Could you check a few things on this model? Use its own coordinates, in mm. A direction names the side the tool comes from. Coordinates: 2 decimals unless noted, no trailing zeros. Loops run counter-clockwise (first coordinate to the right, second up) from the corner with the lowest first, then second, coordinate; pieces in that order, holes last.
1) Thinking about a two-plate mould opening in X: for faces 1 (the face through (-2, 0, -2)), 2 (the face through (4, 2, 0)), 3 (the face through (-0.225, -0.715, 2.24)), which applies, released by +X, released by -X, zero draft, split by the parting line, or undercut?
2) For faces 4 (the face through (13.17, 0.07, 1.5)), 5 (the face through (1, 0, 3)), 6 (the face through (4, -2, 0)), which set-ups out of +Z, -Z, +X, -X, +Y, -Y let a thin tool reach every point of the face, with its end or its side?
3) Will these pins go through, and if not, where does the flat tip stop? P1, Ø1.5, axis at y = -4, z = -0.5, coming from the +X side; P2, Ø1.5, axis at x = 2, z = 0, coming from the +Y side; P3, Ø2.5, axis at x = 3, z = -1, coming from the -Y side; P4, Ø1.5, axis at x = 4, y = -0.5, coming from the +Z side.
4) Imagine slicing it at D-D on x = -0.25. Please give me the cut outline in (y, z).
5) Imagine slicing it at B-B on z = 0. Please give me the cut outline in (x, y).
6) Imagine slicing it at A-A on y = 0. Give the number of separate pieces and of enclosed holes in the cut face, plus the area to 4 significant figures.
7) If I drill on line 1 along Z through (x, y) = (2, 1); line 2 along X through (y, z) = (0, -2.6); line 3 along X through (y, z) = (-3.5, 1), over which ranges is the centre line in solid material (lowest first)?
8) Imagine slicing it at C-C on z = 2.5. Please give me the cut outline in (x, y).
```python
from build123d import *

# Parameters (mm, degrees)
EXTRUDE_1_DEPTH     = 3
SKETCH_2_R          = 5
EXTRUDE_2_DEPTH     = 1.5
SKETCH_3_R          = 3.5
EXTRUDE_3_DEPTH     = 1
SKETCH_4_R          = 1.5
EXTRUDE_4_DEPTH     = 12
SKETCH_5_W          = 10
SKETCH_5_H          = 3
CUT_EXTRUDE_1_DEPTH = 22.313141486
CHAMFER_1_SIZE      = 0.5


with BuildPart() as part:
    # 草图1 → 凸台-拉伸1 (new, symmetric)
    with BuildSketch(Plane.XY):
        with BuildLine():
            Line((5, 2), (0, 2))
            ThreePointArc((0, 2), (1.414213562, 1.414213562), (2, 0))
            ThreePointArc((2, 0), (1.414213562, -1.414213562), (0, -2))
            Line((0, -2), (5, -2))
            Line((5, -2), (5, 2))
        make_face()
        with BuildLine():
            ThreePointArc((2, 0), (1.414213562, 1.414213562), (0, 2))
            Line((0, 2), (0, 0.75))
            ThreePointArc((0, 0.75), (0.530330086, 0.530330086), (0.75, 0))
            ThreePointArc((0.75, 0), (0.530330086, -0.530330086), (0, -0.75))
            Line((0, -0.75), (0, -2))
            ThreePointArc((0, -2), (1.414213562, -1.414213562), (2, 0))
        make_face()
        with BuildLine():
            Line((0, 0.75), (0, 2))
            ThreePointArc((0, 2), (-2, 0), (0, -2))
            Line((0, -2), (0, -0.75))
            ThreePointArc((0, -0.75), (-0.75, 0), (0, 0.75))
        make_face()
    extrude(amount=EXTRUDE_1_DEPTH, both=True)

    # 草图2 → 凸台-拉伸2 (add)
    with BuildSketch(Plane(origin=(5, 0, 0), x_dir=(0, 0, -1), z_dir=(1, 0, 0))):
        Circle(SKETCH_2_R)
    extrude(amount=EXTRUDE_2_DEPTH)

    # 草图3 → 凸台-拉伸3 (add)
    with BuildSketch(Plane(origin=(6.5, 0, 0), x_dir=(0, 0, -1), z_dir=(1, 0, 0))):
        Circle(SKETCH_3_R)
    extrude(amount=EXTRUDE_3_DEPTH)

    # 草图4 → 凸台-拉伸4 (add)
    with BuildSketch(Plane(origin=(7.5, 0, 0), x_dir=(0, 0, -1), z_dir=(1, 0, 0))):
        Circle(SKETCH_4_R)
    extrude(amount=EXTRUDE_4_DEPTH)

    # 草图5 → 切除-拉伸1 (cut, through all)
    with BuildSketch(Plane(origin=(0, 2, 0), x_dir=(1, 0, 0), z_dir=(0, 1, 0))):
        with Locations((-2, 0)):
            Rectangle(SKETCH_5_W, SKETCH_5_H)
    extrude(amount=-CUT_EXTRUDE_1_DEPTH, mode=Mode.SUBTRACT)

    # 倒角1
    chamfer_1_edges = [part.edges().sort_by_distance(p)[0] for p in [
        (19.5, 0, 1.5),
    ]]
    chamfer(chamfer_1_edges, length=CHAMFER_1_SIZE)


solid = part.part
```
Filled in:
1. face 1: released by -X
1. face 2: zero draft
1. face 3: undercut
2. face 4: +X
2. face 5: +Z, -X, +Y, -Y
2. face 6: +Z, -Z, -X, -Y
3. P1: stops at x = 7.5
3. P2: passes through
3. P3: stops at y = -2
3. P4: stops at z = 3
4. outline: (-1.98, -3) - (-0.71, -3) - (-0.71, -1.5) - (-1.98, -1.5) - close; (-1.98, 1.5) - (-0.71, 1.5) - (-0.71, 3) - (-1.98, 3) - close; (0.71, -3) - (1.98, -3) - (1.98, -1.5) - (0.71, -1.5) - close; (0.71, 1.5) - (1.98, 1.5) - (1.98, 3) - (0.71, 3) - close
5. outline: (3, -2) - (5, -2) - (5, -5) - (6.5, -5) - (6.5, -3.5) - (7.5, -3.5) - (7.5, -1.5) - (19, -1.5) - (19.5, -1) - (19.5, 1) - (19, 1.5) - (7.5, 1.5) - (7.5, 3.5) - (6.5, 3.5) - (6.5, 5) - (5, 5) - (5, 2) - (3, 2) - close
6. separate pieces: 3
6. enclosed holes: 0
6. area: 80.25 mm2
7. line 1: z = -3 to -1.5, 1.5 to 3
7. line 2: x = -2 to -0.75, 0.75 to 7.5
7. line 3: x = 5 to 6.5
8. outline: (0, -2) - (5, -2) - (5, -4.33) - (6.5, -4.33) - (6.5, -2.45) - (7.5, -2.45) - (7.5, 2.45) - (6.5, 2.45) - (6.5, 4.33) - (5, 4.33) - (5, 2) - (0, 2) arc R2 ccw to start; hole circle Ø1.5 at (0, 0)
